Source: three-view drawing plus pictorial views. Frame: mm from the lowest corner of the part. A direction names the side the tool comes from. Give positions to 0.01 mm unless a question says otherwise; leave off trailing zeros. Write each loop counter-clockwise with the first axis right and the second up, starting at its lowest first coordinate (ties: lowest second). Pieces come first, ordered by that corner, then holes. Notation, with made-up numbers: M -10,30.25 L 9,30.25 A26 ccw 9,57.25 Z; hole C 27.5,-36.5 d4. An arc over 180 degrees is marked long. Return JSON: item names as keys, results as strings.
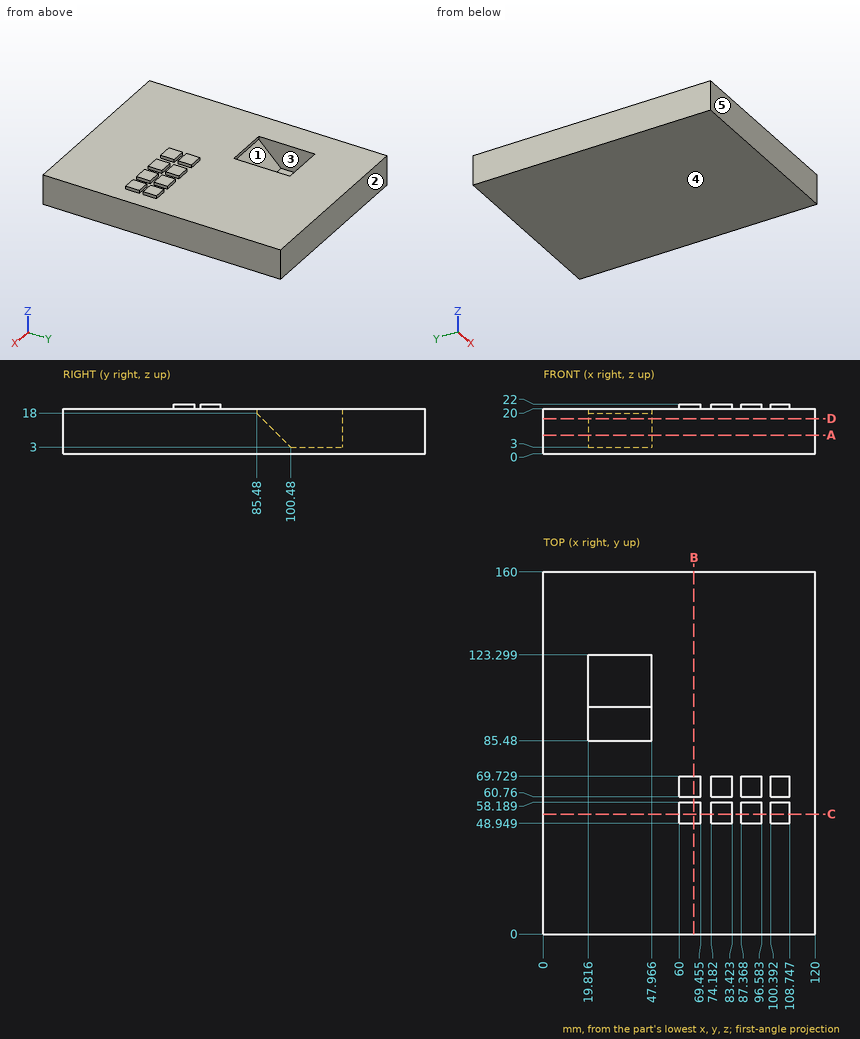
1) Contact query for flat-ended pins moving along their axis: pin 1 Ø1 at (x, z) = (65.5, 21) entering from -Y; pin 2 Ø1.6 at (x, z) = (103, 21) entering from +Y; pin 3 Ø7 at (x, y) = (34, 106.5) entering from +Z. Output: stop coordinate, or through.
Numbers:
{"pin 1": "stops at y = 48.95", "pin 2": "stops at y = 69.73", "pin 3": "stops at z = 3"}
2) Cut plane C-C, the plane y = 53. Return the cut outline in (x, z) (1 decimal), then the cut area to 3 significant figures.
Numbers:
{"outline": "M 0,0 L 120,0 L 120,20 L 108.7,20 L 108.7,22 L 100.4,22 L 100.4,20 L 96.6,20 L 96.6,22 L 87.4,22 L 87.4,20 L 83.4,20 L 83.4,22 L 74.2,22 L 74.2,20 L 69.5,20 L 69.5,22 L 60,22 L 60,20 L 0,20 Z", "area": "2,470 mm²"}
3) Draft query along Y for the marked faces 3, 4 and 5. Return one class per face: released by +Y, released by -Y, zero draft, split by the parting line, or undercut.
Numbers:
{"face 3": "undercut", "face 4": "zero draft", "face 5": "released by -Y"}
4) Set-up query: the marked faces 1 and 2. Return all of +Z, -Z, +X, -X, +Y, -Y with unobstructed straight access to the full face (end or side cutting, diameter ignored); none if empty.
Numbers:
{"face 1": "+Z", "face 2": "+Z, -Z, +X, -X, +Y"}
5) Cut plane B-B, the plane x = 66.5. Return the cut outline in (y, z).
Numbers:
{"outline": "M 0,0 L 160,0 L 160,20 L 69.73,20 L 69.73,22 L 60.76,22 L 60.76,20 L 58.19,20 L 58.19,22 L 48.95,22 L 48.95,20 L 0,20 Z"}
6) Cut plane A-A, the plane z = 8.25. Return the cut outline in (x, y), then the cut area to 3 significant figures.
Numbers:
{"outline": "M 0,0 L 120,0 L 120,160 L 0,160 Z; hole M 19.82,95.23 L 47.97,95.23 L 47.97,123.3 L 19.82,123.3 Z", "area": "18,400 mm²"}
7) Line query: line 1 (X direction, y = 106, z = 14); line 2 (Y direction, x = 41, z = 18.75); line 3 (Z direction, x = 86, y = 123.5). Output: solid intervals per line, ascending. Write a range as [from, to].
Numbers:
{"line 1": "x = [0, 19.82], [47.97, 120]", "line 2": "y = [0, 85.48], [123.3, 160]", "line 3": "z = [0, 20]"}
8) Cut plane D-D, the plane z = 15.5. Return the cut outline in (x, y), then the cut area to 3 significant figures.
Numbers:
{"outline": "M 0,0 L 120,0 L 120,160 L 0,160 Z; hole M 19.82,87.98 L 47.97,87.98 L 47.97,123.3 L 19.82,123.3 Z", "area": "18,200 mm²"}
